Job drawing, mm, ordinate dimensions from the low corner. One solid piece. Give positions to 0.01 mm unless a question says otherwise; leave off trailing zeros. Loops run counter-clockwise (first coordinate to the right, second up) from the corner with the lowest first, then second, coordinate; pieces in that order, holes last. Notation, with made-up numbers: M -6.75,-26 L 24.25,-26 A24 cw 24.25,-13 Z; hole C 44.25,81.25 d5. An arc over 180 degrees is marked long. Answer as CSV lines item,"result".
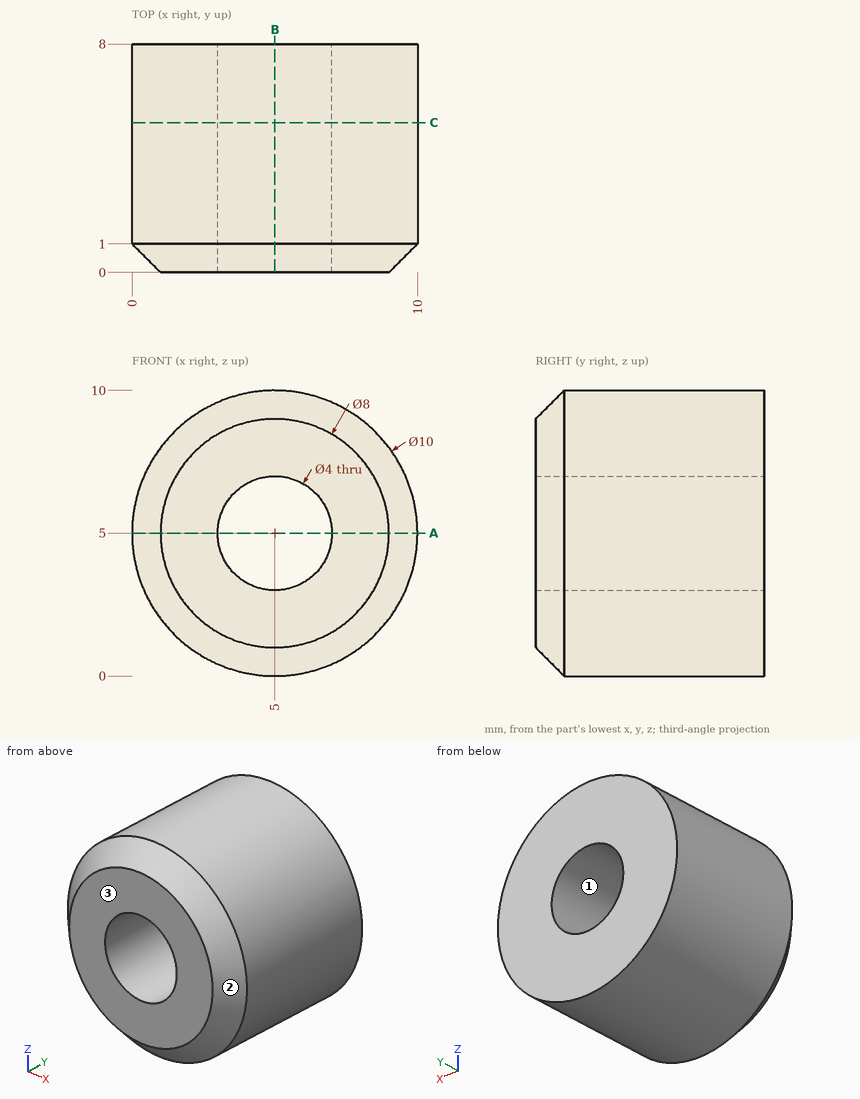
1) Band-saw the part on A-A on z = 5. Give the cut face in (x, y).
Answer below:
outline,"M 0,1 L 1,0 L 3,0 L 3,8 L 0,8 Z; M 7,0 L 9,0 L 10,1 L 10,8 L 7,8 Z"
2) Drill centre lines: line 1 (Z direction, x = 5, y = 5.5); line 2 (X direction, y = 4.5, z = 3.25); line 3 (X direction, y = 1.5, z = 6.25). Where is each one in solid material? Low to high. Write a range as from..to.
Answer below:
line 1,"z = 0..3, 7..10"
line 2,"x = 0.32..4.03, 5.97..9.68"
line 3,"x = 0.16..3.44, 6.56..9.84"
3) Flat gauge pins, fed straight in: pin 1 (2.5 mm diameter, centred on x = 5, z = 5, fed in from +Y); pin 2 (1 mm diameter, centred on y = 5.5, z = 3.5, fed in from -X); pin 3 (2 mm diameter, centred on y = 5, z = 8, fed in from +X); pin 4 (1 mm diameter, centred on y = 4.5, z = 3, fed in from -X). Where does each tip first touch, or does it go through?
Answer below:
pin 1,"passes through"
pin 2,"stops at x = 0.1"
pin 3,"stops at x = 9.58"
pin 4,"stops at x = 0.23"
4) Mould opens along X. For the marked faces 1, 2 and 3 say: +X half, -X half, draft (parallel to the pull), parting line (faces both ways), or undercut.
Answer below:
face 1,"undercut"
face 2,"parting line"
face 3,"draft"
5) Band-saw the part on C-C on y = 5.25. Give the cut face in (x, z).
Answer below:
outline,"C 5,5 d10; hole C 5,5 d4"
6) Band-saw the part on B-B on x = 5. Give the cut face in (y, z).
Answer below:
outline,"M 0,1 L 1,0 L 8,0 L 8,3 L 0,3 Z; M 0,7 L 8,7 L 8,10 L 1,10 L 0,9 Z"
